Design review of the part built by this model. Coordinates are the model's own, in mm. A direction names the side the tool comes from. Coordinates: 2 decimals unless noted, no trailing zeros. Write each loop counter-clockwise with the first axis right and the second up, starting at its lowest first coordinate (ties: lowest second). Pieces come first, ordered by that corner, then holes. Notation, with made-up numbers: M 85.5,51.25 L 139.5,51.25 A6 cw 139.5,58.25 Z; hole C -6,-22.75 d4. An arc over 180 degrees is marked long. Write item = value, one per line.
```python
from build123d import *

# Parameters (mm, degrees)
BOSS_EXTRUDE1_DEPTH = 5
SKETCH2_R           = 2.0125
CUT_EXTRUDE1_DEPTH  = 3
SKETCH3_R           = 2.125
CUT_EXTRUDE2_DEPTH  = 1
SKETCH4_R           = 1
CUT_EXTRUDE3_DEPTH  = 5


with BuildPart() as part:
    # Sketch1 → Boss-Extrude1 (new body)
    with BuildSketch(Plane.XY):
        with BuildLine():
            Line((0, 5), (60, 5))
            ThreePointArc((60, 5), (65, 0), (60, -5))
            Line((60, -5), (0, -5))
            ThreePointArc((0, -5), (-5, 0), (0, 5))
        make_face()
    extrude(amount=BOSS_EXTRUDE1_DEPTH)

    # Sketch2 → Cut-Extrude1 (cut)
    with BuildSketch(Plane(origin=(0, 0, 0), x_dir=(-1, 0, 0), z_dir=(0, 0, -1))):
        Circle(SKETCH2_R)
    extrude(amount=-CUT_EXTRUDE1_DEPTH, mode=Mode.SUBTRACT)

    # Sketch3 → Cut-Extrude2 (cut)
    with BuildSketch(Plane.XY.offset(5)):
        Circle(SKETCH3_R)
    extrude(amount=-CUT_EXTRUDE2_DEPTH, mode=Mode.SUBTRACT)

    # Sketch4 → Cut-Extrude3 (cut, through all)
    with BuildSketch(Plane.XY.offset(4)):
        Circle(SKETCH4_R)
    extrude(amount=-CUT_EXTRUDE3_DEPTH, mode=Mode.SUBTRACT)


solid = part.part
```
Q1. Wall thickness on line 1 (Y direction, x = 0, z = 3.7); line 2 (Y direction, x = 0, z = 2.4); line 3 (X direction, y = 0.25, z = 0.55): over which ranges is each line inside the solid? List them lowest first.
Check result:
line_1 = -5 to -1, 1 to 5
line_2 = -5 to -2.01, 2.01 to 5
line_3 = -4.99 to -2, 2 to 64.99
Q2. Consider section C-C, the plane y = 3.25. State the section outline as (x, z) points.
Check result:
outline = M -3.8,0 L 63.8,0 L 63.8,5 L -3.8,5 Z
Q3. Consider section A-A, the plane y = 0. State the section outline as (x, z) points (1 decimal), and give its area (3 significant figures).
Check result:
outline = M -5,0 L -2,0 L -2,3 L -1,3 L -1,4 L -2.1,4 L -2.1,5 L -5,5 Z; M 1,3 L 2,3 L 2,0 L 65,0 L 65,5 L 2.1,5 L 2.1,4 L 1,4 Z
area = 332 mm²
Q4. Machinability: for faces 4 (the cylindrical face through (-1.92, 0.6, 1.48)), 5 (the flat face through (30, -5, 2)), 6 (the cylindrical face through (1.142, 1.792, 4.507)), which of the approach directions +Z, -Z, +X, -X, +Y, -Y give a long, thin tool a straight path to every point of the face, cutting with its end or side? Answer none if there is none.
Check result:
face_4 = -Z
face_5 = +Z, -Z, +X, -X, -Y
face_6 = +Z
Q5. For P1, Ø1.6, axis at x = 0, y = 0, coming from the +Z side; P2, Ø2, axis at x = -0.5, y = -0.5, coming from the -Z side, all flat-tipped, find the tip position at first contact; note any pin that passes through.
Check result:
P1 = through
P2 = 3
Q6. The part is to be moulded in two halves that separate along X. For faces 1 (the flat face through (30, 0, 5)), 2 (the cylindrical face through (65, 0, 2)), 3 (the cylindrical face through (-0.217, -0.976, 3.507)), say which applies: +X half, -X half, draft (parallel to the pull), parting line (faces both ways), or undercut.
Check result:
face_1 = draft
face_2 = +X half
face_3 = undercut
Q7. Consider section B-B, the plane z = 2.35. State the section outline as (x, y) points (1 decimal).
Check result:
outline = M 0,-5 L 60,-5 A5 ccw 60,5 L 0,5 A5 ccw Z; hole C 0,0 d4
